from build123d import *

# Parameters (mm, degrees)
F0_R      = 127
F1_DEPTH  = 50.8
F2_R      = 88.9
F3_DEPTH  = 1.27
F4_R      = 12.7
F5_DEPTH  = 50.8
F6_R      = 50.8
F7_DEPTH  = 1.27
F8_R      = 88.9
F8_R_2    = 38.1
F9_DEPTH  = 38.1
F10_SIZE  = 7.62
F11_R     = 5.08
F13_DEPTH = 44.45
F14_R     = 30.068591
F14_R_2   = 12.7
F15_DEPTH = 1.27
F17_DEPTH = 44.45
F18_R     = 2.5
F19_DEPTH = 25.4


with BuildPart() as f1:
    # F0 (on Front) → F1 (new body)
    with BuildSketch(Plane.XZ):
        Circle(F0_R)
    extrude(amount=F1_DEPTH)

    # F2 (on face) → F3 (cut)
    with BuildSketch(Plane.XZ.offset(50.8)):
        Circle(F2_R)
    extrude(amount=-F3_DEPTH, mode=Mode.SUBTRACT)

    # F4 (on face) → F5 (cut)
    with BuildSketch(Plane.XZ.offset(49.53)):
        Circle(F4_R)
    extrude(amount=-F5_DEPTH, mode=Mode.SUBTRACT)

    # F6 (on face) → F7 (cut)
    with BuildSketch(Plane.XZ.offset(49.53)):
        Circle(F6_R)
    extrude(amount=-F7_DEPTH, mode=Mode.SUBTRACT)

    # F8 (on face) → F9 (cut)
    with BuildSketch(Plane(origin=(0, 0, 0), x_dir=(-1, 0, 0), z_dir=(0, 1, 0))):
        Circle(F8_R)
        Circle(F8_R_2, mode=Mode.SUBTRACT)
    extrude(amount=-F9_DEPTH, mode=Mode.SUBTRACT)

    # F10
    f10_edges = [f1.edges().sort_by_distance(p)[0] for p in [
        (38.1, -38.1, 0),
    ]]
    chamfer(f10_edges, length=F10_SIZE)

    # F11
    f11_edges = [f1.edges().sort_by_distance(p)[0] for p in [
        (88.9, -38.1, 0),
    ]]
    fillet(f11_edges, radius=F11_R)

    # F12 (on face) → F13 (join)
    with BuildSketch(Plane.XZ.offset(50.8)):
        with BuildLine():
            ThreePointArc((-2.998611, 107.908345), (0, 107.95), (2.998611, 107.908345))
            ThreePointArc((2.998611, 107.908345), (7.602326, 109.70383), (9.525, 114.255894))
            Line((9.525, 114.255894), (9.525, 126.642309))
            ThreePointArc((9.525, 126.642309), (0, 127), (-9.525, 126.642309))
            Line((-9.525, 126.642309), (-9.525, 114.255894))
            ThreePointArc((-9.525, 114.255894), (-7.602326, 109.70383), (-2.998611, 107.908345))
        make_face()
        with BuildLine():
            Line((-74.055926, 87.52631), (-82.814443, 96.284827))
            ThreePointArc((-82.814443, 96.284827), (-89.802561, 89.802561), (-96.284827, 82.814443))
            Line((-96.284827, 82.814443), (-87.52631, 74.055926))
            ThreePointArc((-87.52631, 74.055926), (-82.947979, 72.196666), (-78.42306, 74.182384))
            ThreePointArc((-78.42306, 74.182384), (-76.332177, 76.332177), (-74.182384, 78.42306))
            ThreePointArc((-74.182384, 78.42306), (-72.196666, 82.947979), (-74.055926, 87.52631))
        make_face()
        with BuildLine():
            Line((-114.255894, 9.525), (-126.642309, 9.525))
            ThreePointArc((-126.642309, 9.525), (-127, 0), (-126.642309, -9.525))
            Line((-126.642309, -9.525), (-114.255894, -9.525))
            ThreePointArc((-114.255894, -9.525), (-109.70383, -7.602326), (-107.908345, -2.998611))
            ThreePointArc((-107.908345, -2.998611), (-107.95, 0), (-107.908345, 2.998611))
            ThreePointArc((-107.908345, 2.998611), (-109.70383, 7.602326), (-114.255894, 9.525))
        make_face()
        with BuildLine():
            Line((-87.52631, -74.055926), (-96.284827, -82.814443))
            ThreePointArc((-96.284827, -82.814443), (-89.802561, -89.802561), (-82.814443, -96.284827))
            Line((-82.814443, -96.284827), (-74.055926, -87.52631))
            ThreePointArc((-74.055926, -87.52631), (-72.196666, -82.947979), (-74.182384, -78.42306))
            ThreePointArc((-74.182384, -78.42306), (-76.332177, -76.332177), (-78.42306, -74.182384))
            ThreePointArc((-78.42306, -74.182384), (-82.947979, -72.196666), (-87.52631, -74.055926))
        make_face()
        with BuildLine():
            Line((-9.525, -114.255894), (-9.525, -126.642309))
            ThreePointArc((-9.525, -126.642309), (0, -127), (9.525, -126.642309))
            Line((9.525, -126.642309), (9.525, -114.255894))
            ThreePointArc((9.525, -114.255894), (7.602326, -109.70383), (2.998611, -107.908345))
            ThreePointArc((2.998611, -107.908345), (0, -107.95), (-2.998611, -107.908345))
            ThreePointArc((-2.998611, -107.908345), (-7.602326, -109.70383), (-9.525, -114.255894))
        make_face()
        with BuildLine():
            Line((74.055926, -87.52631), (82.814443, -96.284827))
            ThreePointArc((82.814443, -96.284827), (89.802561, -89.802561), (96.284827, -82.814443))
            Line((96.284827, -82.814443), (87.52631, -74.055926))
            ThreePointArc((87.52631, -74.055926), (82.947979, -72.196666), (78.42306, -74.182384))
            ThreePointArc((78.42306, -74.182384), (76.332177, -76.332177), (74.182384, -78.42306))
            ThreePointArc((74.182384, -78.42306), (72.196666, -82.947979), (74.055926, -87.52631))
        make_face()
        with BuildLine():
            Line((114.255894, -9.525), (126.642309, -9.525))
            ThreePointArc((126.642309, -9.525), (127, 0), (126.642309, 9.525))
            Line((126.642309, 9.525), (114.255894, 9.525))
            ThreePointArc((114.255894, 9.525), (109.70383, 7.602326), (107.908345, 2.998611))
            ThreePointArc((107.908345, 2.998611), (107.95, 0), (107.908345, -2.998611))
            ThreePointArc((107.908345, -2.998611), (109.70383, -7.602326), (114.255894, -9.525))
        make_face()
        with BuildLine():
            Line((87.52631, 74.055926), (96.284827, 82.814443))
            ThreePointArc((96.284827, 82.814443), (89.802561, 89.802561), (82.814443, 96.284827))
            Line((82.814443, 96.284827), (74.055926, 87.52631))
            ThreePointArc((74.055926, 87.52631), (72.196666, 82.947979), (74.182384, 78.42306))
            ThreePointArc((74.182384, 78.42306), (76.332177, 76.332177), (78.42306, 74.182384))
            ThreePointArc((78.42306, 74.182384), (82.947979, 72.196666), (87.52631, 74.055926))
        make_face()
    extrude(amount=-F13_DEPTH)

    # F14 (on face) → F15 (cut)
    with BuildSketch(Plane(origin=(0, 0, 0), x_dir=(-1, 0, 0), z_dir=(0, 1, 0))):
        Circle(F14_R)
        Circle(F14_R_2, mode=Mode.SUBTRACT)
    extrude(amount=-F15_DEPTH, mode=Mode.SUBTRACT)

    # F16 (on face) → F17 (cut)
    with BuildSketch(Plane.XZ.offset(50.8)):
        with BuildLine():
            ThreePointArc((-103.131845, 49.277911), (-98.986704, 57.15), (-94.241845, 64.675843))
            Line((-94.241845, 64.675843), (-105.270432, 71.0432))
            ThreePointArc((-105.270432, 71.0432), (-109.985226, 63.5), (-114.160432, 55.645268))
            Line((-114.160432, 55.645268), (-103.131845, 49.277911))
        make_face()
        with BuildLine():
            ThreePointArc((-94.241845, -64.675843), (-98.986704, -57.15), (-103.131845, -49.277911))
            Line((-103.131845, -49.277911), (-114.160432, -55.645268))
            ThreePointArc((-114.160432, -55.645268), (-109.985226, -63.5), (-105.270432, -71.0432))
            Line((-105.270432, -71.0432), (-94.241845, -64.675843))
        make_face()
        with BuildLine():
            ThreePointArc((8.89, -113.953753), (0, -114.3), (-8.89, -113.953753))
            Line((-8.89, -113.953753), (-8.89, -126.688468))
            ThreePointArc((-8.89, -126.688468), (0, -127), (8.89, -126.688468))
            Line((8.89, -126.688468), (8.89, -113.953753))
        make_face()
        with BuildLine():
            ThreePointArc((103.131845, -49.277911), (98.986704, -57.15), (94.241845, -64.675843))
            Line((94.241845, -64.675843), (105.270432, -71.0432))
            ThreePointArc((105.270432, -71.0432), (109.985226, -63.5), (114.160432, -55.645268))
            Line((114.160432, -55.645268), (103.131845, -49.277911))
        make_face()
        with BuildLine():
            ThreePointArc((94.241845, 64.675843), (98.986704, 57.15), (103.131845, 49.277911))
            Line((103.131845, 49.277911), (114.160432, 55.645268))
            ThreePointArc((114.160432, 55.645268), (109.985226, 63.5), (105.270432, 71.0432))
            Line((105.270432, 71.0432), (94.241845, 64.675843))
        make_face()
        with BuildLine():
            Line((8.89, 113.953753), (8.89, 126.688468))
            ThreePointArc((8.89, 126.688468), (0, 127), (-8.89, 126.688468))
            Line((-8.89, 126.688468), (-8.89, 113.953753))
            ThreePointArc((-8.89, 113.953753), (0, 114.3), (8.89, 113.953753))
        make_face()
    extrude(amount=-F17_DEPTH, mode=Mode.SUBTRACT)

    # F18 (on face) → F19 (cut)
    with BuildSketch(Plane.XZ.offset(6.35)):
        with Locations((0, 120.321111)):
            Circle(F18_R)
        with Locations((-104.201138, 60.160555)):
            Circle(F18_R)
        with Locations((-104.201138, -60.160555)):
            Circle(F18_R)
        with Locations((0, -120.321111)):
            Circle(F18_R)
        with Locations((104.201138, -60.160555)):
            Circle(F18_R)
        with Locations((104.201138, 60.160555)):
            Circle(F18_R)
    extrude(amount=-F19_DEPTH, mode=Mode.SUBTRACT)


solid = f1.part
Work out the finished part from the listing and answer in its coordinate system (mm). A direction names the side the tool comes from. Coordinates: 2 decimals unless noted, no trailing zeros. Write each loop counter-clockwise with the first axis right and the second up, starting at its lowest first coordinate (ties: lowest second). Pieces come first, ordered by that corner, then holes. Notation, with made-up numbers: M 23,24 L 33,24 A22 cw 33,40 Z; hole C 6.25,4 d7. An arc over 180 degrees is marked long. Answer as CSV lines item,"result". Start each with the question number.
Item 1: Section D-D on z = 110 is taken. Write down the section's boundary in (x, y).
Item 2: Consider L1, parallel to Z at x = -20, y = -34; L2, parallel to Z at x = -38, y = -37; L3, parallel to Z at x = -5, y = -40.5. Determine where each line is inside the solid, lowest interval first.
Item 3: Determine the mould class of faces 4 (the face through (8.89, -29, 120)), 5 (the face through (100, -29, -68)), 6 (the face through (-127, -29, 0)) for opening direction Z: released by +Z, released by -Z, zero draft, split by the parting line, or undercut.
Item 4: Flat-ended cylindrical pins translate along their axes: P1, Ø5, axis at x = -57, z = 35, coming from the -Y side; P2, Ø6, axis at x = -19, y = -24.5, coming from the -Z side; P3, Ø2, axis at x = 71, z = 1.5, coming from the +Y side; P4, Ø14.5, axis at x = -3, z = 119, coming from the -Y side. Find the tip coordinate at first contact, or state that the pin passes through.
Item 5: Section A-A on y = -15 is taken. Give the number of separate pieces and of enclosed holes in the cut face, and give its area (3 significant figures).
Item 6: A tool of negligible diameter and unlimited length cuts with its end or side. For faces 1 (the face through (-100, -29, -68)), 2 (the face through (108.723, -28.886, -52.506)), 3 (the face through (-0.1, -28.9, 114.3)), from which of +Z, -Z, +X, -X, +Y, -Y can it reach the whole face along a straight path? Write none if from no direction.
Checks:
1,outline,"M -63.47,-50.8 L 63.47,-50.8 L 63.47,0 L -63.47,0 Z"
2,L1,"z = -125.42 to -86.52, -36.5 to 36.5, 86.52 to 125.42"
2,L2,"z = -121.18 to -78.24, -23.39 to 23.39, 78.24 to 121.18"
2,L3,"z = -114.19 to -11.67, 11.67 to 114.19"
3,face 4,"zero draft"
3,face 5,"undercut"
3,face 6,"split by the parting line"
4,P1,"stops at y = -49.53"
4,P2,"stops at z = -125.99"
4,P3,"stops at y = -38.1"
4,P4,"stops at y = -50.8"
5,separate pieces,"2"
5,enclosed holes,"2"
5,area,"28,500 mm²"
6,face 1,"-X, -Y"
6,face 2,"-Y"
6,face 3,"+Z, -Y"
